Autodesk Inventor part; units mm, degrees
ref_plane "YZ Plane" through (0, 0, 0) normal (1, 0, 0) x (0, 1, 0)
ref_plane "XZ Plane" through (0, 0, 0) normal (0, 1, 0) x (-1, 0, 0)
ref_plane "XY Plane" through (0, 0, 0) normal (0, 0, 1) x (1, 0, 0)
sketch "Sketch1" plane through (0, 0, 0) normal (0, 0, 1) x (1, 0, 0)
  circle A0 centre (0, 0) radius 2.5
  circle A1 centre (0, 0) radius 5
  dimension "d0" = 10
extrude "Extrusion1" add sketch "Sketch1" against normal blind 14
sketch "Sketch2" plane through (0, 0, -14) normal (0, 0, -1) x (-1, 0, 0)
  circle A0 centre (0, 0) radius 7.5
  dimension "d3" = 15
extrude "Extrusion2" add sketch "Sketch2" against normal blind 8
properties part number "Gear_ele"
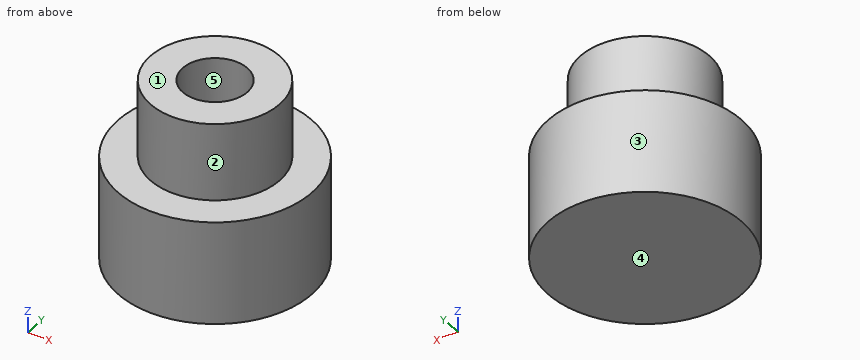
Could you check a few things on this model? Use its own coordinates, in mm. Face numbers are marked on the shaded views. A direction names the side the tool comes from. Round coordinates to 2 decimals unless told otherwise and drop trailing zeros. Write each loop counter-clockwise with the first axis right and the second up, starting at its lowest first coordinate (ties: lowest second). Pieces come first, ordered by that corner, then holes. Notation, with made-up numbers: M -21,69 L 3,69 A16 cw 3,81 Z; hole C 11.25,36.25 d1. An arc over 180 degrees is marked long. Answer in a Markdown table with one row per item. Add a question column.
Q1. On a 3-axis mill with a long thin cutter (end or side, diameter ignored), from which of +Z, -Z, +X, -X, +Y, -Y can I reach the whole of each face in a straight line? I mean the marked faces 1 and 2. Say none if no direction works.
Q2. Imagine slicing it at D-D (z = -12.25). Please give me the cut outline in (x, y).
Q3. Imagine slicing it at C-C (z = -3.75). Please give me the cut outline in (x, y).
Q4. Imagine slicing it at A-A (y = 0). Please give me the cut outline in (x, z).
Q5. Will these pins go through, and if not, where does the flat tip stop? pin 1 Ø4 at (x, y) = (0, 0) entering from +Z; pin 2 Ø1 at (x, z) = (-2, -6.5) entering from +Y.
Q6. If we mould it in two halves opening along X, with no side actions, what happens to the marked faces 3, 4 and 5? For each: +X half, -X half, draft (parallel to the pull), parting line (faces both ways), or undercut.
Q7. If I drill on line 1 (Y direction, x = 0, z = -3.05); line 2 (Z direction, x = 6.25, y = -2.25); line 3 (X direction, y = 0.5, z = -4.25), over which ranges is the centre line in solid material (lowest first)? Write a range as from..to.
Values:
| question | item | result |
|---|---|---|
| 1 | face 1 | +Z, +X, -X, +Y, -Y |
| 1 | face 2 | +Z |
| 2 | outline | C 0,0 d15 |
| 3 | outline | C 0,0 d10; hole C 0,0 d5 |
| 4 | outline | M -7.5,-14 L 7.5,-14 L 7.5,-6 L 5,-6 L 5,0 L 2.5,0 L 2.5,-6 L -2.5,-6 L -2.5,0 L -5,0 L -5,-6 L -7.5,-6 Z |
| 5 | pin 1 | z = -6 |
| 5 | pin 2 | y = 7.35 |
| 6 | face 3 | parting line |
| 6 | face 4 | draft |
| 6 | face 5 | undercut |
| 7 | line 1 | -5..-2.5, 2.5..5 |
| 7 | line 2 | -14..-6 |
| 7 | line 3 | -4.97..-2.45, 2.45..4.97 |
